The model under review builds one solid part; all positions refer to its coordinate system, in mm. A direction names the side the tool comes from. Round coordinates to 2 decimals unless told otherwise and drop trailing zeros. Order: outer loops, then holes, each group sorted by start corner. A loop starts at its lowest first (then second) coordinate and runs counter-clockwise, first axis right, second up.
```python
from build123d import *

# Parameters (mm, degrees)
F1_DEPTH = 100
F3_DEPTH = 182


with BuildPart() as f1:
    # F0 (on Front) → F1 (new body)
    with BuildSketch(Plane.XZ):
        Polygon((0, 150), (0, 0), (100, 0), (100, 20), (60, 150), (40, 150), (40, 140), (20, 140), (20, 150), align=None)
    extrude(amount=F1_DEPTH)

    # F2 (on face) → F3 (cut)
    with BuildSketch(Plane.XY.offset(150)):
        Polygon((140, -60), (140, -50), (140, -40), (49.901433, -40), (49.901433, -60), align=None)
    extrude(amount=-F3_DEPTH, mode=Mode.SUBTRACT)


solid = f1.part
```
(1) Insertion check: pin 1 (16 mm diameter, centred on y = -54, z = 72.5, fed in from +X); pin 2 (5 mm diameter, centred on y = -27.5, z = 147.5, fed in from +X); pin 3 (5 mm diameter, centred on y = -63.5, z = 40, fed in from +X). Each pin has a flat end and moves straight along its axis. Give the tip position at first contact, or say it passes through.
Data:
pin 1: stops at x = 85.47
pin 2: stops at x = 61.54
pin 3: stops at x = 94.62
(2) Consider section A-A (x = 85). Write out the cut boundary in (y, z).
Data:
outline: (-100, 0) - (-60, 0) - (-60, 68.75) - (-100, 68.75) - close; (-40, 0) - (0, 0) - (0, 68.75) - (-40, 68.75) - close
(3) For faces 5 (the flat face through (70, -40, 59)), 6 (the flat face through (30, -49, 140)), 7 (the flat face through (80.28, -19.72, 84.09)), list the 3-axis set-ups (+Z, -Z, +X, -X, +Y, -Y) from which the entire face can be reached by the end or side of a thin tool; tool diameter is ignored.
Data:
face 5: +Z, -Z, +X
face 6: +Z, +Y, -Y
face 7: +Z, +X, +Y, -Y
(4) Draft analysis for pull direction Y (two halves, no side actions). For faces 1 (the flat face through (38, 0, 76)), 2 (the flat face through (49.901, -50, 76)), 3 (the flat face through (69, -60, 59)), 4 (the flat face through (40, -49, 145)), state which applies: pulls with the +Y half, pulls with the -Y half, needs draft (parallel to the pull), parting line crosses it, or undercut.
Data:
face 1: pulls with the +Y half
face 2: undercut
face 3: undercut
face 4: needs draft
(5) Consider section B-B (y = -44). Write out the cut boundary in (x, z), and give its area (3 significant figures).
Data:
outline: (0, 0) - (49.9, 0) - (49.9, 150) - (40, 150) - (40, 140) - (20, 140) - (20, 150) - (0, 150) - close
area: 7,290 mm2
(6) Consider section D-D (x = 74). Write out the cut boundary in (y, z).
Data:
outline: (-100, 0) - (-60, 0) - (-60, 104.5) - (-100, 104.5) - close; (-40, 0) - (0, 0) - (0, 104.5) - (-40, 104.5) - close
(7) To check wall thickness, follow probe 1 along Y at (x, z) = (70, 49); probe 2 along X at (y, z) = (-53.5, 141); probe 3 along X at (y, z) = (-46, 101.5). State the ranges of each line that lie inside material, in increasing order.
Data:
probe 1: y = -100 to -60, -40 to 0
probe 2: x = 0 to 20, 40 to 49.9
probe 3: x = 0 to 49.9
(8) Consider section C-C (z = 124). Write out the cut boundary in (x, y), and give its area (3 significant figures).
Data:
outline: (0, -100) - (68, -100) - (68, -60) - (49.9, -60) - (49.9, -40) - (68, -40) - (68, 0) - (0, 0) - close
area: 6,440 mm2
